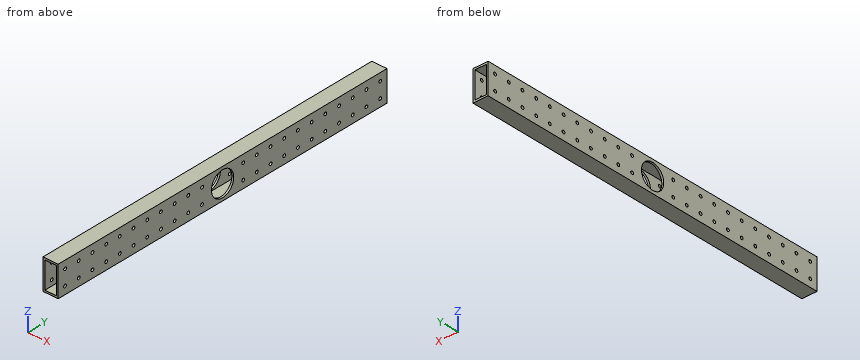
from build123d import *

# Parameters (mm, degrees)
F0_W     = 25.4
F0_H     = 50.8
F0_W_2   = 19.05
F0_H_2   = 44.45
F1_DEPTH = 609.6
F2_R     = 2.5527
F3_DEPTH = 25.4
F4_R     = 20.6375
F5_DEPTH = 25.4


with BuildPart() as f1:
    # F0 (on Front) → F1 (new body)
    with BuildSketch(Plane.XZ):
        Rectangle(F0_W, F0_H)
        Rectangle(F0_W_2, F0_H_2, mode=Mode.SUBTRACT)
    extrude(amount=F1_DEPTH)

    # F2 (on face) → F3 (cut)
    with BuildSketch(Plane.YZ.offset(12.7)):
        with Locations((-596.9, 12.7)):
            Circle(F2_R)
        with Locations((-596.9, -12.7)):
            Circle(F2_R)
        with Locations((-571.5, 12.7)):
            Circle(F2_R)
        with Locations((-571.5, -12.7)):
            Circle(F2_R)
        with Locations((-546.1, 12.7)):
            Circle(F2_R)
        with Locations((-546.1, -12.7)):
            Circle(F2_R)
        with Locations((-520.7, 12.7)):
            Circle(F2_R)
        with Locations((-520.7, -12.7)):
            Circle(F2_R)
        with Locations((-495.3, 12.7)):
            Circle(F2_R)
        with Locations((-495.3, -12.7)):
            Circle(F2_R)
        with Locations((-469.9, 12.7)):
            Circle(F2_R)
        with Locations((-469.9, -12.7)):
            Circle(F2_R)
        with Locations((-444.5, 12.7)):
            Circle(F2_R)
        with Locations((-444.5, -12.7)):
            Circle(F2_R)
        with Locations((-419.1, 12.7)):
            Circle(F2_R)
        with Locations((-419.1, -12.7)):
            Circle(F2_R)
        with Locations((-393.7, 12.7)):
            Circle(F2_R)
        with Locations((-393.7, -12.7)):
            Circle(F2_R)
        with Locations((-368.3, 12.7)):
            Circle(F2_R)
        with Locations((-368.3, -12.7)):
            Circle(F2_R)
        with Locations((-342.9, 12.7)):
            Circle(F2_R)
        with Locations((-342.9, -12.7)):
            Circle(F2_R)
        with Locations((-317.5, 12.7)):
            Circle(F2_R)
        with Locations((-317.5, -12.7)):
            Circle(F2_R)
        with Locations((-292.1, 12.7)):
            Circle(F2_R)
        with Locations((-292.1, -12.7)):
            Circle(F2_R)
        with Locations((-266.7, 12.7)):
            Circle(F2_R)
        with Locations((-266.7, -12.7)):
            Circle(F2_R)
        with Locations((-241.3, 12.7)):
            Circle(F2_R)
        with Locations((-241.3, -12.7)):
            Circle(F2_R)
        with Locations((-215.9, 12.7)):
            Circle(F2_R)
        with Locations((-215.9, -12.7)):
            Circle(F2_R)
        with Locations((-190.5, 12.7)):
            Circle(F2_R)
        with Locations((-190.5, -12.7)):
            Circle(F2_R)
        with Locations((-165.1, 12.7)):
            Circle(F2_R)
        with Locations((-165.1, -12.7)):
            Circle(F2_R)
        with Locations((-139.7, 12.7)):
            Circle(F2_R)
        with Locations((-139.7, -12.7)):
            Circle(F2_R)
        with Locations((-114.3, 12.7)):
            Circle(F2_R)
        with Locations((-114.3, -12.7)):
            Circle(F2_R)
        with Locations((-88.9, 12.7)):
            Circle(F2_R)
        with Locations((-88.9, -12.7)):
            Circle(F2_R)
        with Locations((-63.5, 12.7)):
            Circle(F2_R)
        with Locations((-63.5, -12.7)):
            Circle(F2_R)
        with Locations((-38.1, 12.7)):
            Circle(F2_R)
        with Locations((-38.1, -12.7)):
            Circle(F2_R)
        with Locations((-12.7, 12.7)):
            Circle(F2_R)
        with Locations((-12.7, -12.7)):
            Circle(F2_R)
    extrude(amount=-F3_DEPTH, mode=Mode.SUBTRACT)

    # F4 (on face) → F5 (cut)
    with BuildSketch(Plane.YZ.offset(12.7)):
        with Locations((-304.8, 0)):
            Circle(F4_R)
    extrude(amount=-F5_DEPTH, mode=Mode.SUBTRACT)


solid = f1.part
Verification items for the finished model (mm, model axes). Give positions to 0.01 mm unless a question says otherwise; leave off trailing zeros. Write each loop counter-clockwise with the first axis right and the second up, starting at its lowest first coordinate (ties: lowest second). Pieces come first, ordered by that corner, then holes. Notation, with made-up numbers: M -26,-1.75 L 33,-1.75 A16 ccw 33,6.25 Z; hole C 3.25,27.5 d3. An arc over 180 degrees is marked long. Put each result on its own line as item: value. Start each with the question number.
1. Section check B-B (x = 5.25). Record the cut outline in (y, z) (3 decimals).
2. Scan lines: line 1 along Z through (x, y) = (-11.4, -393.7); line 2 along Z through (x, y) = (-8.5, -272) (3 decimals); line 3 along X through (y, z) = (-152, -6) (3 decimals). Record each from-to range of solid material in increasing order. Write a range as [from, to].
3. Section check A-A (y = -353). Record the cut outline in (x, z) (3 decimals).
Answer list:
1. outline: M -609.6,-25.4 L 0,-25.4 L 0,-22.225 L -609.6,-22.225 Z; M -609.6,22.225 L 0,22.225 L 0,25.4 L -609.6,25.4 Z
2. line 1: [-25.4, -15.25], [-10.15, 10.15], [15.25, 25.4]
2. line 2: [-25.4, -22.225], [22.225, 25.4]
2. line 3: [-12.7, -9.525], [9.525, 12.7]
3. outline: M -12.7,-25.4 L 12.7,-25.4 L 12.7,25.4 L -12.7,25.4 Z; hole M -9.525,-22.225 L 9.525,-22.225 L 9.525,22.225 L -9.525,22.225 Z
